from build123d import *

# Parameters (mm, degrees)
CROQUIS1_W               = 72
CROQUIS1_H               = 74
SALIENTE_EXTRUIR3_DEPTH  = 4
CROQUIS2_W               = 3
CROQUIS2_H               = 6
SALIENTE_EXTRUIR4_DEPTH  = 7.6
CORTAR_EXTRUIR3_DEPTH    = 83.938591741
CROQUIS5_W               = 5
CROQUIS5_H               = 4
SALIENTE_EXTRUIR5_DEPTH  = 1
CROQUIS9_W               = 72
CROQUIS9_H               = 1.5
SALIENTE_EXTRUIR6_DEPTH  = 8
CROQUIS10_W              = 72
CROQUIS10_H              = 5.9
SALIENTE_EXTRUIR7_DEPTH  = 2
CROQUIS11_W              = 10
CROQUIS11_H              = 4.4
SALIENTE_EXTRUIR10_DEPTH = 7
SALIENTE_EXTRUIR14_DEPTH = 10
CROQUIS15_W              = 18
CROQUIS15_H              = 4.4
SALIENTE_EXTRUIR15_DEPTH = 5
CROQUIS16_W              = 72
CROQUIS16_H              = 40
SALIENTE_EXTRUIR16_DEPTH = 10.5
CROQUIS17_W              = 72
CROQUIS17_H              = 5
SALIENTE_EXTRUIR17_DEPTH = 8
CROQUIS18_W              = 72
CROQUIS18_H              = 8
SALIENTE_EXTRUIR19_DEPTH = 2
CROQUIS19_W              = 72
CROQUIS19_H              = 1
CORTAR_EXTRUIR4_DEPTH    = 14.5
CROQUIS20_W              = 56
CROQUIS20_H              = 7
SALIENTE_EXTRUIR20_DEPTH = 65
CORTAR_EXTRUIR6_REACH    = 103.4
CROQUIS27_W              = 56
CROQUIS27_H              = 9
CROQUIS26_R              = 1.25
CROQUIS26_R_2            = 1.3
CORTAR_EXTRUIR8_DEPTH    = 10


with BuildPart() as part:
    # Croquis1 → Saliente-Extruir3 (new body)
    with BuildSketch(Plane.XY):
        with Locations((0, -2.5)):
            Rectangle(CROQUIS1_W, CROQUIS1_H)
    extrude(amount=SALIENTE_EXTRUIR3_DEPTH)

    # Croquis2 → Saliente-Extruir4 (add)
    with BuildSketch(Plane.XY.offset(4)):
        with Locations((-34.5, -36.5)):
            Rectangle(CROQUIS2_W, CROQUIS2_H)
        with Locations((34.5, -36.5)):
            Rectangle(CROQUIS2_W, CROQUIS2_H)
    extrude(amount=SALIENTE_EXTRUIR4_DEPTH)

    # Croquis3 → Cortar-Extruir3 (cut, through all)
    with BuildSketch(Plane.ZY.offset(36)):
        Polygon((4, -39.5), (11.6, -36.5), (11.6, -39.5), align=None)
    extrude(amount=-CORTAR_EXTRUIR3_DEPTH, mode=Mode.SUBTRACT)

    # Croquis5 → Saliente-Extruir5 (add)
    with BuildSketch(Plane.XY.offset(4)):
        with Locations((-33.5, -30.5)):
            Rectangle(CROQUIS5_W, CROQUIS5_H)
        with Locations((33.5, -29.5)):
            Rectangle(CROQUIS5_W, CROQUIS5_H)
    extrude(amount=SALIENTE_EXTRUIR5_DEPTH)

    # Croquis9 → Saliente-Extruir6 (add)
    with BuildSketch(Plane.XY.offset(4)):
        with Locations((0, -26.35)):
            Rectangle(CROQUIS9_W, CROQUIS9_H)
    extrude(amount=SALIENTE_EXTRUIR6_DEPTH)

    # Croquis10 → Saliente-Extruir7 (add)
    with BuildSketch(Plane.XY.offset(12)):
        with Locations((0, -28.55)):
            Rectangle(CROQUIS10_W, CROQUIS10_H)
    extrude(amount=SALIENTE_EXTRUIR7_DEPTH)

    # Croquis11 → Saliente-Extruir10 (add)
    with BuildSketch(Plane.XY.offset(14)):
        with Locations((-31, -29.3)):
            Rectangle(CROQUIS11_W, CROQUIS11_H)
        with Locations((31, -29.3)):
            Rectangle(CROQUIS11_W, CROQUIS11_H)
    extrude(amount=-SALIENTE_EXTRUIR10_DEPTH)

    # Croquis14 → Saliente-Extruir14 (add)
    with BuildSketch(Plane.XY.offset(4)):
        with BuildLine():
            Line((-9, -23.7), (-9, -25.6))
            Line((-9, -25.6), (-2.1, -25.6))
            ThreePointArc((-2.1, -25.6), (-2.656497116, -24.256497116), (-4, -23.7))
            Line((-4, -23.7), (-9, -23.7))
        make_face()
        with BuildLine():
            Line((-9, -21.2), (-9, -22.2))
            Line((-9, -22.2), (-4, -22.2))
            ThreePointArc((-4, -22.2), (-2.22447191, -22.714955647), (-1, -24.1))
            Line((-1, -24.1), (1, -24.1))
            ThreePointArc((1, -24.1), (2.22447191, -22.714955647), (4, -22.2))
            Line((4, -22.2), (9, -22.2))
            Line((9, -22.2), (9, -21.2))
            Line((9, -21.2), (-9, -21.2))
        make_face()
        with BuildLine():
            ThreePointArc((4, -23.7), (2.656497116, -24.256497116), (2.1, -25.6))
            Line((2.1, -25.6), (9, -25.6))
            Line((9, -25.6), (9, -23.7))
            Line((9, -23.7), (4, -23.7))
        make_face()
    extrude(amount=SALIENTE_EXTRUIR14_DEPTH)

    # Croquis15 → Saliente-Extruir15 (add)
    with BuildSketch(Plane.XY.offset(4)):
        with Locations((0, -23.4)):
            Rectangle(CROQUIS15_W, CROQUIS15_H)
    extrude(amount=SALIENTE_EXTRUIR15_DEPTH)

    # Croquis16 → Saliente-Extruir16 (add)
    with BuildSketch(Plane.XY.offset(4)):
        with Locations((0, 14.5)):
            Rectangle(CROQUIS16_W, CROQUIS16_H)
    extrude(amount=SALIENTE_EXTRUIR16_DEPTH)

    # Croquis17 → Saliente-Extruir17 (add)
    with BuildSketch(Plane.XY.offset(14.5)):
        with Locations((0, 32)):
            Rectangle(CROQUIS17_W, CROQUIS17_H)
    extrude(amount=SALIENTE_EXTRUIR17_DEPTH)

    # Croquis18 → Saliente-Extruir19 (add)
    with BuildSketch(Plane(origin=(0, 34.5, 0), x_dir=(1, 0, 0), z_dir=(0, 1, 0))):
        with Locations((0, -18.5)):
            Rectangle(CROQUIS18_W, CROQUIS18_H)
    extrude(amount=SALIENTE_EXTRUIR19_DEPTH)

    # Croquis19 → Cortar-Extruir4 (cut)
    with BuildSketch(Plane(origin=(0, 0, 0), x_dir=(-1, 0, 0), z_dir=(0, 0, -1))):
        with Locations((0, 34)):
            Rectangle(CROQUIS19_W, CROQUIS19_H)
    extrude(amount=-CORTAR_EXTRUIR4_DEPTH, mode=Mode.SUBTRACT)

    # Croquis20 → Saliente-Extruir20 (add)
    with BuildSketch(Plane(origin=(0, 0, 0), x_dir=(-1, 0, 0), z_dir=(0, 0, -1))):
        with Locations((0, -36)):
            Rectangle(CROQUIS20_W, CROQUIS20_H)
    extrude(amount=SALIENTE_EXTRUIR20_DEPTH)

    # Croquis27 → Cortar-Extruir6 (cut, up to next)
    with BuildSketch(Plane(origin=(0, -32.5, 0), x_dir=(1, 0, 0), z_dir=(0, 1, 0)), mode=Mode.PRIVATE) as cortar_extruir6_sk1:
        with Locations((0, 60.5)):
            Rectangle(CROQUIS27_W, CROQUIS27_H)
    cortar_extruir6_tool1 = extrude(cortar_extruir6_sk1.sketch, amount=-CORTAR_EXTRUIR6_REACH, mode=Mode.PRIVATE) & part.part
    add(cortar_extruir6_tool1.solids().sort_by_distance((0, -32.5, -60.5))[0], mode=Mode.SUBTRACT)

    # Croquis26 → Cortar-Extruir8 (cut)
    with BuildSketch(Plane(origin=(0, -32.5, 0), x_dir=(1, 0, 0), z_dir=(0, 1, 0))):
        with Locations(Location((-18, 5, 0), (0, 0, 270))):
            Circle(CROQUIS26_R)
        with Locations(Location((18, 5, 0), (0, 0, 270))):
            Circle(CROQUIS26_R)
        with Locations(Location((-23, 43.25, 0), (0, 0, 270))):
            Circle(CROQUIS26_R)
        with Locations(Location((-24, 5, 0), (0, 0, 270))):
            Circle(CROQUIS26_R_2)
        Polygon((18.5, 53.25), (-20.5, 53.25), (-20.5, 33.25), (-10.5, 33.25), (-10.5, 7.5), (25.5, 7.5), (25.5, 32.5), (18.5, 32.5), align=None)
        with Locations(Location((24, 5, 0), (0, 0, 270))):
            Circle(CROQUIS26_R_2)
    extrude(amount=-CORTAR_EXTRUIR8_DEPTH, mode=Mode.SUBTRACT)


solid = part.part
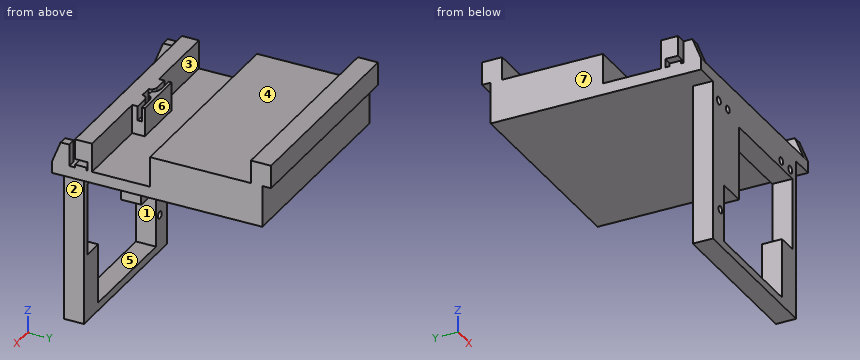
The model under review builds one solid part; all positions refer to its coordinate system, in mm. Face numbers are marked on the shaded views. A direction names the side the tool comes from. Round coordinates to 2 decimals unless told otherwise and drop trailing zeros. Write each loop counter-clockwise with the first axis right and the second up, starting at its lowest first coordinate (ties: lowest second). Pieces come first, ordered by that corner, then holes. Notation, with made-up numbers: M -24,-31 L -4,-31 A21 ccw -4,-15 Z; hole C 81.5,81.25 d11. An arc over 180 degrees is marked long. Use a Markdown table: item, result. Add a question column.
Q1. To check wall thickness, follow line 1 (X direction, y = -35, z = -5); line 2 (X direction, y = -37.5, z = -43.25); line 3 (X direction, y = -33.5, z = -28). State the ranges of each line that lie inside material, in increasing order.
Q2. Insertion check: pin 1 (3.5 mm diameter, centred on x = 0.5, y = -30, fed in from -Z); pin 2 (2 mm diameter, centred on x = -34.5, y = -30.5, fed in from +Z); pin 3 (1 mm diameter, centred on x = 5.5, y = -3.5, fed in from +Z); pin 4 (12 mm diameter, centred on y = -23, z = -40.5, fed in from -X). Each pin has a flat end and moves straight along its axis. Give the tip position at first contact, or say it passes through.
Q3. We need section B-B, the plane z = -43.25. State the section outline as (x, y) points, plus the area to 4 significant figures.
Q4. The part is to be moulded in two halves that separate along X. For the marked faces 5, 6 and 7, say which applies: pulls with the +X half, pulls with the -X half, needs draft (parallel to the pull), parting line crosses it, or undercut.
Q5. Machinability: for the marked faces 1, 2, 3 and 4, which of the approach directions +Z, -Z, +X, -X, +Y, -Y give a long, thin tool a straight path to every point of the face, cutting with its end or side? Answer none if there is none.
Q6. We need section D-D, the plane x = 24. State the section outline as (y, z) points.
Q7. We need section C-C, the plane z = -13. State the section outline as (x, y) points.
Q8. We need section A-A, the plane x = -18. State the section outline as (y, z) points, plus the area to 3 significant figures.
Findings below:
| question | item | result |
|---|---|---|
| 1 | line 1 | x = -28 to -25.3, -22.7 to -19.25, -16.75 to 16.75, 19.25 to 22.7, 25.3 to 28 |
| 1 | line 2 | x = -28 to -24.25, -21.75 to -20.5, 18.5 to 28 |
| 1 | line 3 | x = -28 to -10.5, 25.5 to 28 |
| 2 | pin 1 | stops at z = 0 |
| 2 | pin 2 | stops at z = 14 |
| 2 | pin 3 | stops at z = 14.5 |
| 2 | pin 4 | passes through |
| 3 | outline | M -28,-39.5 L -24.25,-39.5 L -24.25,-32.5 L -28,-32.5 Z; M -21.75,-39.5 L -20.5,-39.5 L -20.5,-32.5 L -21.75,-32.5 Z; M 18.5,-39.5 L 28,-39.5 L 28,-32.5 L 18.5,-32.5 Z |
| 3 | area | 101.5 mm² |
| 4 | face 5 | undercut |
| 4 | face 6 | needs draft |
| 4 | face 7 | pulls with the -X half |
| 5 | face 1 | +Y, -Y |
| 5 | face 2 | -Z, +X, +Y, -Y |
| 5 | face 3 | +Z, -X |
| 5 | face 4 | +Z, +X, -X, -Y |
| 6 | outline | M -39.5,-56 L -32.5,-56 L -32.5,-32.5 L -39.5,-32.5 Z; M -39.5,-7.5 L -32.5,-7.5 L -32.5,-6.3 L -39.5,-6.3 Z; M -39.5,-3.7 L -32.5,-3.7 L -32.5,0 L 33.5,0 L 33.5,14.5 L 36.5,14.5 L 36.5,22.5 L 29.5,22.5 L 29.5,14.5 L -5.5,14.5 L -5.5,4 L -25.6,4 L -25.6,14 L -31.5,14 L -31.5,12 L -27.1,12 L -27.1,4 L -39.5,4 Z |
| 7 | outline | M -28,-39.5 L -10.5,-39.5 L -10.5,-32.5 L -28,-32.5 Z; M 25.5,-39.5 L 28,-39.5 L 28,-32.5 L 25.5,-32.5 Z |
| 8 | outline | M -39.5,-56 L -32.5,-56 L -32.5,-53.25 L -39.5,-53.25 Z; M -39.5,-33.25 L -32.5,-33.25 L -32.5,-6.25 L -39.5,-6.25 Z; M -39.5,-3.75 L -32.5,-3.75 L -32.5,0 L 33.5,0 L 33.5,14.5 L 36.5,14.5 L 36.5,22.5 L 29.5,22.5 L 29.5,14.5 L -5.5,14.5 L -5.5,4 L -25.6,4 L -25.6,14 L -31.5,14 L -31.5,12 L -27.1,12 L -27.1,4 L -39.5,4 Z |
| 8 | area | 1,020 mm² |
